The model under review builds one solid part; all positions refer to its coordinate system, in mm. Face numbers are marked on the shaded views. A direction names the side the tool comes from. Round coordinates to 2 decimals unless told otherwise and drop trailing zeros. Order: outer loops, then holes, each group sorted by start corner. A loop starts at its lowest first (then second) coordinate and runs counter-clockwise, first axis right, second up. Notation, with made-up numbers: M 47.5,42 L 60.5,42 A23 cw 60.5,57 Z; hole C 51,49.5 d8. An arc over 180 degrees is marked long. Answer as a JSON object with one key per item and string values. Group by question number.
1) For the marked faces 5 and 6, list the 3-axis set-ups (+Z, -Z, +X, -X, +Y, -Y) from which the entire face can be reached by the end or side of a thin tool; tool diameter is ignored.
2) To check wall thickness, follow line 1 (X direction, y = 8.5, z = 16.5); line 2 (Y direction, x = -2, z = 24.5) (3 decimals); line 3 (Z direction, x = 52, y = 74.5). State the ranges of each line that lie inside material, in increasing order.
3) The part is to be moulded in two halves that separate along X. For the marked faces 1, 2, 3 and 4, say which applies: +X half, -X half, draft (parallel to the pull), parting line (faces both ways), or undercut.
4) Insertion check: pin 1 Ø8 at (x, z) = (78, -35) entering from +Y (3 decimals); pin 2 Ø12 at (x, y) = (-12.5, 64.5) entering from -Z. Each pin has a flat end and moves straight along its axis. Give the tip position at first contact, or say it passes through.
5) Consider section B-B, the plane z = -19. Write out the cut boundary in (x, y) (3 decimals), then the cut area to 3 significant figures.
6) Consider section C-C, the plane x = -98.5. Write out the cut boundary in (y, z) (3 decimals).
7) Consider section A-A, the plane y = 37. Write out the cut boundary in (x, z).
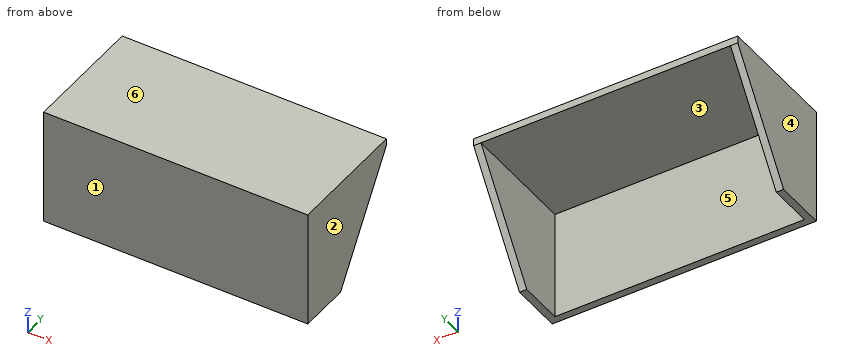
```python
from build123d import *

# Parameters (mm, degrees)
BOSS_EXTRUDE1_DEPTH     = 115
SKETCH2_R               = 2.5
CUT_EXTRUDE1_DEPTH      = 171.92584101
CUT_EXTRUDE2_DEPTH      = 150.015569656
CUT_EXTRUDE2_DEPTH_BACK = 150.015569656
SKETCH4_R               = 3.3
SPLIT1_SURFACE_1_BACK   = 266.855
SPLIT1_SURFACE_1_DEPTH  = 533.71
SPLIT1_SURFACE_2_BACK   = 266.855
SPLIT1_SURFACE_2_DEPTH  = 533.71
SKETCH6_W               = 6.35
SKETCH6_H               = 21.6
BOSS_EXTRUDE2_DEPTH     = 230
DELETEFACE1_START       = -3.175
DELETEFACE1_OUTLINE_R   = 3.3
DELETEFACE1_DEPTH       = 6.35
DELETEFACE1_START_2     = 44.45
DELETEFACE1_2_OUTLINE_R = 2.5
DELETEFACE1_2_DEPTH     = 6.35
BOSS_EXTRUDE3_DEPTH     = 6.35


# Read off the part's stored shape, not the designer's step: DeleteFace1
with BuildPart() as part:
    # Sketch1 → Boss-Extrude1 (new, symmetric)
    with BuildSketch(Plane(origin=(0, 0, 0), x_dir=(0, 0, -1), z_dir=(1, 0, 0))):
        Polygon((-50.8, -3.175), (50.8, -3.175), (50.8, 3.175), (-44.45, 3.175), (-44.45, 83.175), (-50.8, 83.175), (-50.8, 3.175), align=None)
    extrude(amount=BOSS_EXTRUDE1_DEPTH, both=True)

    # Sketch2 → Cut-Extrude1 (cut, through all)
    with BuildSketch(Plane(origin=(0, 0, 44.45), x_dir=(-1, 0, 0), z_dir=(0, 0, -1))):
        with Locations(Location((-32.5, 73.491666667, 0), (0, 0, 90))):
            Circle(SKETCH2_R)
        with Locations(Location((-32.5, 11.825, 0), (0, 0, 90))):
            Circle(SKETCH2_R)
        with Locations(Location((32.5, 11.825, 0), (0, 0, 90))):
            Circle(SKETCH2_R)
        with Locations(Location((32.5, 73.491666667, 0), (0, 0, 90))):
            Circle(SKETCH2_R)
        with Locations(Location((-102.75, 73.491666667, 0), (0, 0, 90))):
            Circle(SKETCH2_R)
        with Locations(Location((-102.75, 11.825, 0), (0, 0, 90))):
            Circle(SKETCH2_R)
        with Locations(Location((102.75, 73.491666667, 0), (0, 0, 90))):
            Circle(SKETCH2_R)
        with Locations(Location((102.75, 11.825, 0), (0, 0, 90))):
            Circle(SKETCH2_R)
    extrude(amount=-CUT_EXTRUDE1_DEPTH, mode=Mode.SUBTRACT)

    # Sketch4 → Cut-Extrude2 (cut, two sides: drawn at the far end of the back side and taken through both)
    with BuildSketch(Plane(origin=(0, 3.175, 0), x_dir=(1, 0, 0), z_dir=(0, 1, 0)).offset(-CUT_EXTRUDE2_DEPTH_BACK)):
        with Locations(Location((56.37, 25.8, 0), (0, 0, 270))):
            Circle(SKETCH4_R)
        with Locations(Location((96.37, 25.8, 0), (0, 0, 270))):
            Circle(SKETCH4_R)
        with Locations(Location((96.37, -27.2, 0), (0, 0, 270))):
            Circle(SKETCH4_R)
        with Locations(Location((56.37, -27.2, 0), (0, 0, 270))):
            Circle(SKETCH4_R)
        with Locations(Location((-96.37, 25.8, 0), (0, 0, 90))):
            Circle(SKETCH4_R)
        with Locations(Location((-96.37, -27.2, 0), (0, 0, 90))):
            Circle(SKETCH4_R)
        with Locations(Location((-56.37, -27.2, 0), (0, 0, 90))):
            Circle(SKETCH4_R)
        with Locations(Location((-56.37, 25.8, 0), (0, 0, 90))):
            Circle(SKETCH4_R)
    extrude(amount=CUT_EXTRUDE2_DEPTH + CUT_EXTRUDE2_DEPTH_BACK, mode=Mode.SUBTRACT)


with BuildPart() as body_2:
    # Split1: the piece behind the surface
    add(part.part)
    # Split1 surface: a surface, the sketch's curves swept straight by 533.71 mm
    with BuildLine(Plane.ZY.offset(115).offset(-SPLIT1_SURFACE_1_BACK), mode=Mode.PRIVATE) as split1_surface_1_path:
        Line((44.45, 3.175), (50.8, 3.175))
    split1_surface_1 = Shell.extrude(split1_surface_1_path.wire(), (-1 * SPLIT1_SURFACE_1_DEPTH, 0 * SPLIT1_SURFACE_1_DEPTH, 0 * SPLIT1_SURFACE_1_DEPTH))
    split(bisect_by=split1_surface_1, keep=Keep.BOTTOM)


with BuildPart() as part_1:
    add(part.part)

    # Split1: split by a surface, the side it looks to stays
    # Split1 surface: a surface, the sketch's curves swept straight by 533.71 mm
    with BuildLine(Plane.ZY.offset(115).offset(-SPLIT1_SURFACE_2_BACK), mode=Mode.PRIVATE) as split1_surface_2_path:
        Line((44.45, 3.175), (50.8, 3.175))
    split1_surface_2 = Shell.extrude(split1_surface_2_path.wire(), (-1 * SPLIT1_SURFACE_2_DEPTH, 0 * SPLIT1_SURFACE_2_DEPTH, 0 * SPLIT1_SURFACE_2_DEPTH))
    split(bisect_by=split1_surface_2, keep=Keep.TOP)

    # Sketch6 → Boss-Extrude2 (add)
    with BuildSketch(Plane.ZY.offset(115)):
        with Locations((47.625, 93.975)):
            Rectangle(SKETCH6_W, SKETCH6_H)
    extrude(amount=-BOSS_EXTRUDE2_DEPTH)


with BuildPart() as body_2_1:
    add(body_2.part)

    # Combine1: union part
    add(part_1.part)

    # DeleteFace1 outline → DeleteFace1 (add)
    with BuildSketch(Plane(origin=(0, 0, 0), x_dir=(1, 0, 0), z_dir=(0, 1, 0)).offset(DELETEFACE1_START)):
        with Locations((56.37, 25.8)):
            Circle(DELETEFACE1_OUTLINE_R)
        with Locations((-56.37, 25.8)):
            Circle(DELETEFACE1_OUTLINE_R)
        with Locations((-56.37, -27.2)):
            Circle(DELETEFACE1_OUTLINE_R)
        with Locations((-96.37, -27.2)):
            Circle(DELETEFACE1_OUTLINE_R)
        with Locations((-96.37, 25.8)):
            Circle(DELETEFACE1_OUTLINE_R)
        with Locations((56.37, -27.2)):
            Circle(DELETEFACE1_OUTLINE_R)
        with Locations((96.37, -27.2)):
            Circle(DELETEFACE1_OUTLINE_R)
        with Locations((96.37, 25.8)):
            Circle(DELETEFACE1_OUTLINE_R)
    extrude(amount=DELETEFACE1_DEPTH)

    # DeleteFace1 2 outline → DeleteFace1 2 (add)
    with BuildSketch(Plane.XY.offset(DELETEFACE1_START_2)):
        with Locations((32.5, 11.825)):
            Circle(DELETEFACE1_2_OUTLINE_R)
        with Locations((-32.5, 11.825)):
            Circle(DELETEFACE1_2_OUTLINE_R)
        with Locations((-32.5, 73.491666667)):
            Circle(DELETEFACE1_2_OUTLINE_R)
        with Locations((102.75, 73.491666667)):
            Circle(DELETEFACE1_2_OUTLINE_R)
        with Locations((-102.75, 11.825)):
            Circle(DELETEFACE1_2_OUTLINE_R)
        with Locations((-102.75, 73.491666667)):
            Circle(DELETEFACE1_2_OUTLINE_R)
        with Locations((102.75, 11.825)):
            Circle(DELETEFACE1_2_OUTLINE_R)
        with Locations((32.5, 73.491666667)):
            Circle(DELETEFACE1_2_OUTLINE_R)
    extrude(amount=DELETEFACE1_2_DEPTH)

    # Sketch10 → Boss-Extrude3 (add)
    with BuildSketch(Plane.ZY.offset(115)):
        Polygon((44.45, 104.775), (-50.8, 41.802895791), (-50.8, 3.175), (44.45, 3.175), align=None)
    boss_extrude3 = extrude(amount=-BOSS_EXTRUDE3_DEPTH)

    # Mirror1: Boss-Extrude3 across plane
    add(boss_extrude3.mirror(Plane(origin=(0, 0, 0), x_dir=(0, 0, 1), z_dir=(1, 0, 0))))


solid = body_2_1.part
```
Results list:
{
 "1": {"face 5": "-Z, +Y", "face 6": "+Z, +X, -X, +Y, -Y"},
 "2": {"line 1": "-115 to -108.65, 108.65 to 115", "line 2": "-3.175 to 3.175", "line 3": "44.45 to 50.8"},
 "3": {"face 1": "draft", "face 2": "+X half", "face 3": "undercut", "face 4": "-X half"},
 "4": {"pin 1": "y = 3.175", "pin 2": "z = 44.45"},
 "5": {"outline": "M -115,-3.175 L 115,-3.175 L 115,62.827 L 108.65,62.827 L 108.65,3.175 L -108.65,3.175 L -108.65,62.827 L -115,62.827 Z", "area": "2,220 mm^2"},
 "6": {"outline": "M -3.175,-50.8 L 3.175,-50.8 L 3.175,44.45 L 104.775,44.45 L 104.775,50.8 L -3.175,50.8 Z"},
 "7": {"outline": "M -115,-50.8 L -108.65,-50.8 L -108.65,44.45 L 108.65,44.45 L 108.65,-50.8 L 115,-50.8 L 115,50.8 L -115,50.8 Z"}
}
